Geometry: see drawing. Coordinates: mm, zero at the bounding-box minimum. A direction names the side the tool comes from. Give positions to 0.01 mm unless a question says otherwise; leave off trailing zeros. Loops run counter-clockwise (first coordinate to the right, second up) from the corner with the lowest first, then second, coordinate; pieces in that order, holes last. Notation, with made-up numbers: (-33, 54) -> (-20, 54) arc R30 ccw to (-20, 90) -> close; hole circle Ø2 at (81.5, -29). An arc over 180 degrees is marked (long way). Return JSON: item names as keys, results as strings. Group by question number.
(1) Ray query, line 1 (X direction, y = 1.75, z = 19.75); line 2 (X direction, y = 1.4, z = 11); line 3 (Z direction, x = 11.75, y = 1.2). Return the intervals inside material, ascending. Write a range as from..to.
(2) Cut plane B-B on z = 17.25. Return loops of the section in (x, y), then the cut area to 3 significant figures.
(3) Cut plane A-A on x = 15. Return loops of the section in (y, z), then the cut area to 3 significant figures.
(4) Draft query along X for the marked faces 3, 4, 5 and 6. Return one class per face: released by +X, released by -X, zero draft, split by the parting line, or undercut.
(5) Cut plane D-D on z = 12.5. Return loops of the section in (x, y), then the cut area to 3 significant figures.
(6) Cut plane C-C on y = 2. Return loops of the section in (x, z) (3 decimals), then the cut area to 3 significant figures.
(7) Access query for the marked faces 1 and 2. Directions: +Z, -Z, +X, -X, +Y, -Y. A direction counts if a zero-diameter tool reaches every point of the face in a straight line with its end or side. Return the directions, or none.
(8) Pin query (flat end, axial travel): pin 1 (0.8 mm diameter, centred on x = 16.5, y = 1, fed in from +Z); pin 2 (1.5 mm diameter, centred on x = 12, y = 1, fed in from +Z); pin 3 (1.5 mm diameter, centred on x = 22.5, z = 14, fed in from -Y); pin 4 (1 mm diameter, centred on x = 4.5, y = 1.5, fed in from -Z). Return the tip coordinate at first contact, or that it passes through.
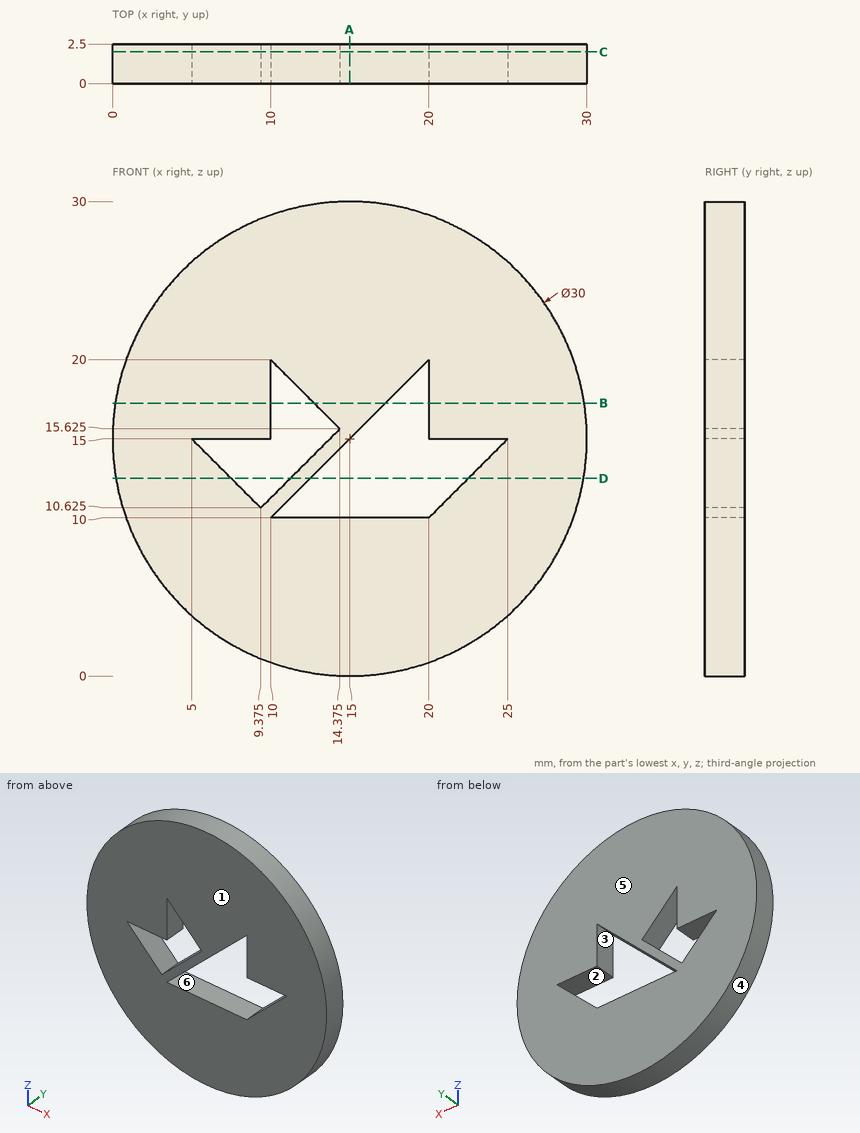
Answers:
{
 "1": {"line 1": "0.77..10, 10.25..19.75, 20..29.23", "line 2": "0.54..9, 9.75..11, 21..29.46", "line 3": "0.36..10, 11.75..13, 18.25..29.64"},
 "2": {"outline": "(0.17, 0) -> (10, 0) -> (10, 2.5) -> (0.17, 2.5) -> close; (12.75, 0) -> (17.25, 0) -> (17.25, 2.5) -> (12.75, 2.5) -> close; (20, 0) -> (29.83, 0) -> (29.83, 2.5) -> (20, 2.5) -> close", "area": "60.4 mm²"},
 "3": {"outline": "(0, 0) -> (2.5, 0) -> (2.5, 10) -> (0, 10) -> close; (0, 15) -> (2.5, 15) -> (2.5, 30) -> (0, 30) -> close", "area": "62.5 mm²"},
 "4": {"face 3": "undercut", "face 4": "split by the parting line", "face 5": "zero draft", "face 6": "undercut"},
 "5": {"outline": "(0.21, 0) -> (7.5, 0) -> (7.5, 2.5) -> (0.21, 2.5) -> close; (11.25, 0) -> (12.5, 0) -> (12.5, 2.5) -> (11.25, 2.5) -> close; (22.5, 0) -> (29.79, 0) -> (29.79, 2.5) -> (22.5, 2.5) -> close", "area": "39.6 mm²"},
 "6": {"outline": "circle Ø30 at (15, 15); hole (5, 15) -> (9.375, 10.625) -> (14.375, 15.625) -> (10, 20) -> (10, 15) -> close; hole (10, 10) -> (20, 10) -> (25, 15) -> (20, 15) -> (20, 20) -> close", "area": "613 mm²"},
 "7": {"face 1": "+Z, -Z, +X, -X, -Y", "face 2": "+Y, -Y"},
 "8": {"pin 1": "z = 29.96", "pin 2": "z = 29.83", "pin 3": "through", "pin 4": "z = 3.82"}
}
